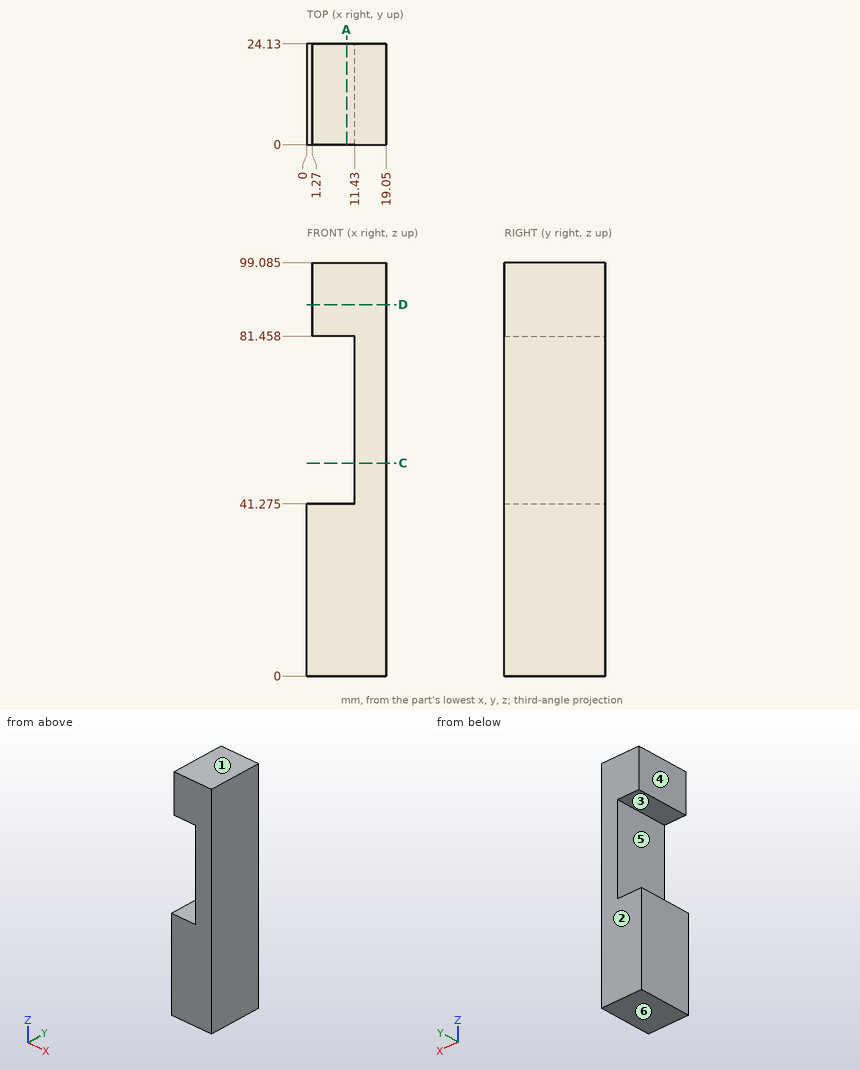
Study the drawing (mm; zero at the part's minimum x, y, z) and answer. A direction names the side the tool comes from. Give positions to 0.01 mm unless a question says otherwise; leave off trailing zeros. Write each loop counter-clockwise with the first axis right and the second up, starting at its lowest first coordinate (ties: lowest second). Pieces come first, ordered by that corner, then holes. Notation, with made-up numbers: M 48,23 L 80,23 A20 cw 80,55 Z; hole C 37.5,82.5 d10. An arc over 180 degrees is marked long. Put each result on its own line as item: value. Start each with the question number.
1. Which of the six approach directions +Z, -Z, +X, -X, +Y, -Y give full straight-line access (tool end or side, diameter ignored) to the marked faces 4, 5 and 6?
2. Consider line 1 along Z through (x, y) = (6.25, 12.5) (1 decimal); line 2 along X through (y, z) = (20.25, 87); line 3 along X through (y, z) = (10.75, 46). Determine where each line is inside the solid, lowest interval first.
3. The part is cut by section C-C, the plane z = 51. Give the vertices of the cut face in (x, y).
4. The part is cut by section D-D, the plane z = 89. Give the vertices of the cut face in (x, y), and give its area (3 significant figures).
5. For a pull along Z with two mould halves and no side action, classify the marked faces 1, 2 and 3 as released by +Z, released by -Z, zero draft, split by the parting line, or undercut.
6. The part is cut by section A-A, the plane x = 9.5. Give the vertices of the cut face in (y, z) (1 decimal).
7. Each of these flat-tipped pins is pushed along its axis until it touches: pin 1 Ø12 at (y, z) = (11, 63) entering from -X; pin 2 Ø5.5 at (y, z) = (9.5, 87.5) entering from -X. Where does it stop, or does it pass through?
Final values:
1. face 4: +Z, -X, +Y, -Y
1. face 5: -X, +Y, -Y
1. face 6: -Z, +X, -X, +Y, -Y
2. line 1: z = 0 to 41.3, 81.5 to 99.1
2. line 2: x = 1.27 to 19.05
2. line 3: x = 11.43 to 19.05
3. outline: M 11.43,0 L 19.05,0 L 19.05,24.13 L 11.43,24.13 Z
4. outline: M 1.27,0 L 19.05,0 L 19.05,24.13 L 1.27,24.13 Z
4. area: 429 mm²
5. face 1: released by +Z
5. face 2: zero draft
5. face 3: undercut
6. outline: M 0,0 L 24.1,0 L 24.1,41.3 L 0,41.3 Z; M 0,81.5 L 24.1,81.5 L 24.1,99.1 L 0,99.1 Z
7. pin 1: stops at x = 11.43
7. pin 2: stops at x = 1.27
